Geometry: see drawing. Coordinates: mm, zero at the bounding-box minimum. A direction names the side the tool comes from. Coordinates: 2 decimals unless noted, no trailing zeros. Order: outer loops, then holes, each group sorted by start corner. A loop starts at its lowest first (then second) coordinate and runs counter-clockwise, first axis right, second up. Notation, with made-up numbers: (-12, 14) -> (18, 14) arc R6 ccw to (18, 20) -> close; hole circle Ø3 at (2.25, -33). An arc over 180 degrees is marked (long way). Write each question's results on one line, items separated by ' | '.
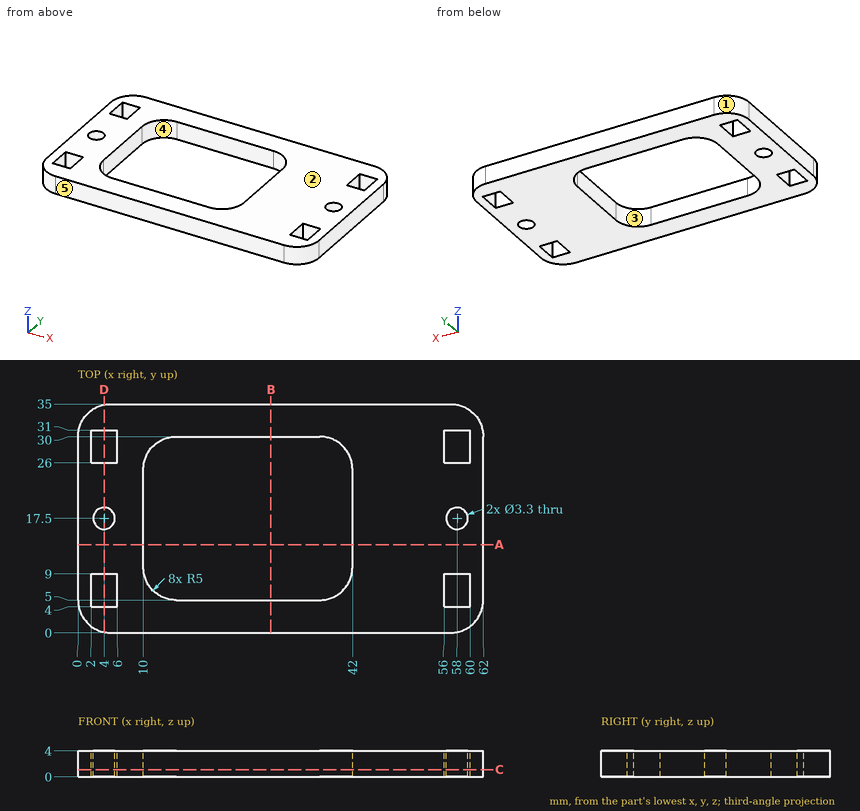
(1) Cut plane A-A, the plane y = 13.5. Return loops of the section in (x, z), plus the area to 3 significant figures.
Return value:
outline: (0, 0) -> (10, 0) -> (10, 4) -> (0, 4) -> close; (42, 0) -> (62, 0) -> (62, 4) -> (42, 4) -> close | area: 120 mm2
(2) Mould query, pull axis Y, two halves, no side actions, for the marked faces 1, 2 and 3. Classes: +Y half, -Y half, draft (parallel to the pull), parting line (faces both ways), or undercut.
Return value:
face 1: +Y half | face 2: draft | face 3: undercut
(3) Reachability of the marked faces 4 and 5 from +Z, -Z, +X, -X, +Y, -Y: full face, straight path, thin tool, end or side. Return the list, or none.
Return value:
face 4: +Z, -Z | face 5: +Z, -Z, +X, -X, -Y
(4) Cut plane C-C, the plane z = 1.1. Count the separate pieces of the cut face and the enclosed holes in it, plus the area to 3 significant figures.
Return value:
separate pieces: 1 | enclosed holes: 7 | area: 1,270 mm2
(5) Cut plane B-B, the plane x = 29.5. Return loops of the section in (y, z), plus the area to 3 significant figures.
Return value:
outline: (0, 0) -> (5, 0) -> (5, 4) -> (0, 4) -> close; (30, 0) -> (35, 0) -> (35, 4) -> (30, 4) -> close | area: 40.0 mm2
(6) Cut plane D-D, the plane x = 4. Return loops of the section in (y, z), plus the area to 3 significant figures.
Return value:
outline: (0.1, 0) -> (4, 0) -> (4, 4) -> (0.1, 4) -> close; (9, 0) -> (15.85, 0) -> (15.85, 4) -> (9, 4) -> close; (19.15, 0) -> (26, 0) -> (26, 4) -> (19.15, 4) -> close; (31, 0) -> (34.9, 0) -> (34.9, 4) -> (31, 4) -> close | area: 86.0 mm2
(7) Line query: line 1 along X through (y, z) = (17.5, 3.05); line 2 along Y through (x, z) = (18.5, 2.95); line 3 along X through (y, z) = (6, 3.4). Output: solid intervals per line, ascending. Write a range as from..to.
Return value:
line 1: 0..2.35, 5.65..10, 42..56.35, 59.65..62 | line 2: 0..5, 30..35 | line 3: 0..2, 6..12, 40..56, 60..62
(8) Pin query (flat end, axial travel): P1, Ø1.2, axis at x = 59, z = 2.5, coming from the +Y side. Return the tip coordinate at first contact, or that it passes through.
Return value:
P1: y = 34.8
